from build123d import *

# Parameters (mm, degrees)
F2_R          = 250
F2_R_2        = 192
F3_DEPTH      = 10
F3_DEPTH_BACK = 5
F5_R          = 20
F7_R          = 25.25
F8_DEPTH      = 5
F10_DEPTH     = 5
F11_R         = 12.5
F12_DEPTH     = 20
F13_R         = 200
F14_DEPTH     = 5


with BuildPart() as f1:
    # F0 (on Front) → F1 (revolve)
    with BuildSketch(Plane.XZ):
        with BuildLine():
            Line((200, 20), (200, 0))
            Line((200, 0), (203, 0))
            Line((203, 0), (203, 20))
            ThreePointArc((203, 20), (196.5493669363, 42.6526770285), (179.1328476019, 58.5088839444))
            ThreePointArc((179.1328476019, 58.5088839444), (92.0009441475, 89.9153591058), (0, 100.6000003082))
            Line((0, 100.6000003082), (0, 97.6))
            ThreePointArc((0, 97.6), (91.3153782925, 86.994742746), (177.7979977692, 55.8222176227))
            ThreePointArc((177.7979977692, 55.8222176227), (193.9994111035, 41.072257701), (200, 20))
        make_face()
    revolve(axis=Axis((0, 0, 99.1000001541), (0, 0, 1)))

    # F2 (on face) → F3 (join, two sides)
    with BuildSketch(Plane(origin=(0, 0, 0), x_dir=(1, 0, 0), z_dir=(0, 0, -1))) as f3_sk:
        Circle(F2_R)
        Circle(F2_R_2, mode=Mode.SUBTRACT)
    extrude(amount=F3_DEPTH)
    extrude(f3_sk.sketch, amount=-F3_DEPTH_BACK)

    # F5 (on offset) → F6 (join, up to the next surface of F1)
    with BuildSketch(Plane.XY.offset(150)):
        Circle(F5_R)
    extrude(until=Until.NEXT, dir=(0, 0, -1))

    # F7 (on face) → F8 (join)
    with BuildSketch(Plane.XY.offset(150)):
        Circle(F7_R)
    extrude(amount=F8_DEPTH)

    # F9 (on face) → F10 (join)
    with BuildSketch(Plane.XY.offset(155)):
        Polygon((-14.1421356237, 14.1421356237), (0, 0), (14.1421356237, 14.1421356237), align=None)
    extrude(amount=F10_DEPTH)

    # F11 (on face) → F12 (cut)
    with BuildSketch(Plane.XY.offset(5)):
        with Locations((227.5, 0)):
            Circle(F11_R)
        with Locations((0, 227.5)):
            Circle(F11_R)
        with Locations((-227.5, 0)):
            Circle(F11_R)
        with Locations((0, -227.5)):
            Circle(F11_R)
    extrude(amount=-F12_DEPTH, mode=Mode.SUBTRACT)

    # F13 (on face) → F14 (cut)
    with BuildSketch(Plane(origin=(0, 0, -10), x_dir=(1, 0, 0), z_dir=(0, 0, -1))):
        Circle(F13_R)
    extrude(amount=-F14_DEPTH, mode=Mode.SUBTRACT)


solid = f1.part
Read the model definition and answer for the solid it produces. Units are mm, in the model's axes. A direction names the side the tool comes from. Give positions to 0.01 mm unless a question says otherwise; leave off trailing zeros. Loops run counter-clockwise (first coordinate to the right, second up) from the corner with the lowest first, then second, coordinate; pieces in that order, holes last. Notation, with made-up numbers: M 25.25,72.5 L 67.25,72.5 A19 ccw 67.25,77.5 Z; hole C 59.5,65.5 d6. An arc over 180 degrees is marked long. Write each question's results on one line, items separated by ' | '.
1. Given pin 1 (5 mm diameter, centred on x = -153.5, z = 41.5, fed in from +Y); pin 2 (22.5 mm diameter, centred on x = 0, y = 227.5, fed in from +Z); pin 3 (25 mm diameter, centred on x = -12, y = -7.5, fed in from +Z); pin 4 (2.5 mm diameter, centred on x = -1, z = 157, fed in from +Y), each flat-ended and moving along its own axis, determine where each tip first touches the part or whether it passes through.
Values:
pin 1: stops at y = 127.59 | pin 2: passes through | pin 3: stops at z = 155 | pin 4: stops at y = 14.14
2. Straight lines are drawn through the part: line 1 (Y direction, x = 0, z = 0); line 2 (Y direction, x = 0, z = -6); line 3 (X direction, y = -108, z = 50). For each, find the intervals that lie inside material, in ascending order. Write a range as [from, to].
Values:
line 1: y = [-250, -240], [-215, -192], [192, 215], [240, 250] | line 2: y = [-250, -240], [-215, -200], [200, 215], [240, 250] | line 3: x = [-157.3, -151.99], [151.99, 157.3]
3. Section C-C on z = 117 is taken. Give the vertices of the cut face in (x, y), plus the area to 3 significant figures.
Values:
outline: C 0,0 d40 | area: 1,260 mm^2
4. The mould has two halves that part along X. Classify faces 1 (the face through (-4.336, -19.524, 125.397)), 2 (the face through (-75, -186, -10)), 3 (the face through (-191.814, -8.442, 0.07)): pulls with the +X half, pulls with the -X half, needs draft (parallel to the pull), parting line crosses it, or undercut.
Values:
face 1: parting line crosses it | face 2: needs draft | face 3: undercut
5. A tool of negligible diameter and unlimited length cuts with its end or side. For faces 4 (the face through (-5.47, -24.65, 152.46)), 5 (the face through (-75, -179, -5)), 6 (the face through (-8, 19, 150)), 7 (the face through (-7, 7, 157)), 8 (the face through (7, 7, 157)), from which of +Z, -Z, +X, -X, +Y, -Y can it reach the whole face along a straight path? Write none if from no direction.
Values:
face 4: +Z | face 5: -Z | face 6: none | face 7: +Z, -X, -Y | face 8: +Z, +X, -Y
6. Section A-A on x = -227.5 is taken. Give the vertices of the cut face in (y, z), plus the area to 3 significant figures.
Values:
outline: M -103.65,-10 L -12.5,-10 L -12.5,5 L -103.65,5 Z; M 12.5,-10 L 103.65,-10 L 103.65,5 L 12.5,5 Z | area: 2,730 mm^2
